CAD build for the part. Positions are in the model's coordinates, mm. Face numbers are marked on the shaded views. Give positions to 0.01 mm unless a question says otherwise; leave off trailing zeros. Loops run counter-clockwise (first coordinate to the right, second up) from the corner with the lowest first, then second, coordinate; pieces in that order, holes last.
Item 1: Drop flat-ended pins along their axis: P1, Ø1.5, axis at x = 9.5, y = 11, coming from the -Z side; P2, Ø4, axis at x = 17, z = 43.5, coming from the +Y side; P3, Ø8, axis at x = 14.5, y = 1, coming from the -Z side; P4, Ø7.5, axis at y = -19.19, z = -12.33, coming from the +X side. Give the stop position or say it passes through.
Item 2: Probe probe 1 along Z at (x, y) = (7, -18); probe 2 along Z at (x, y) = (2.75, -24) (3 decimals); probe 3 along Y at (x, z) = (15.5, -9). List the from-to ranges inside material, lowest first.
Item 3: Mould opens along Z. For the marked faces 1, 2, 3 and 4 say: released by +Z, released by -Z, zero draft, split by the parting line, or undercut.
Item 4: Saw through at B-B on x = 6. Give the cut face in (y, z).
Item 5: Saw through at A-A on z = 63. Give the cut face in (x, y).
Item 6: Saw through at C-C on y = -20.5. Give the cut face in (x, z), plus the area to 3 significant figures.
Item 7: Saw through at D-D on z = -11. Give the cut face in (x, y), plus the area to 3 significant figures.
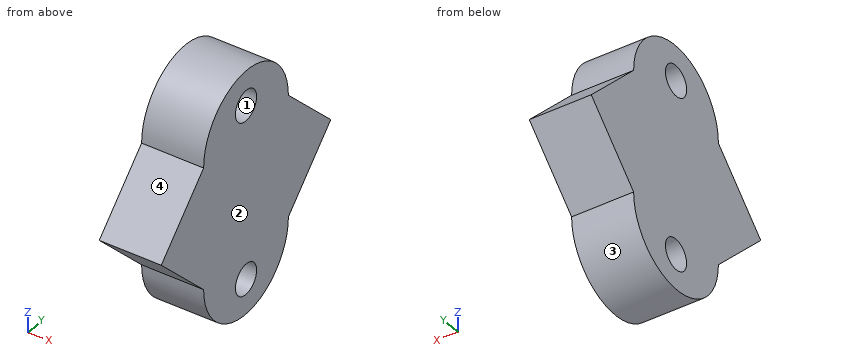
from build123d import *

# Parameters (mm, degrees)
F0_W     = 50.8
F0_H     = 50.8
F1_DEPTH = 25.4
F3_D     = 12.7


with BuildPart() as f1:
    # F0 (on Right) → F1 (new body)
    with BuildSketch(Plane.YZ):
        with BuildLine():
            ThreePointArc((6.2123674129, 49.3127632231), (-19.1876325871, 74.7127632231), (-44.5876325871, 49.3127632231))
            Line((-44.5876325871, 49.3127632231), (6.2123674129, 49.3127632231))
        make_face()
        with Locations((-19.1876325871, 23.9127632231)):
            Rectangle(F0_W, F0_H)
        Polygon((-44.5876325871, -1.4872367769), (-44.5876325871, 49.3127632231), (-69.9876325871, 23.9127632231), align=None)
        Polygon((31.6123674129, 23.9127632231), (6.2123674129, 49.3127632231), (6.2123674129, -1.4872367769), align=None)
        with BuildLine():
            Line((6.2123674129, -1.4872367769), (-44.5876325871, -1.4872367769))
            ThreePointArc((-44.5876325871, -1.4872367769), (-19.1876325871, -26.8872367769), (6.2123674129, -1.4872367769))
        make_face()
    extrude(amount=F1_DEPTH)

    # F3 (through all)
    with Locations(Plane.YZ.offset(25.4)):
        with Locations((-19.1876325871, 60.1578950882), (-19.1876325871, -12.3323686421)):
            Hole(F3_D / 2)


solid = f1.part
Results below:
1. P1: stops at z = 2.55
1. P2: stops at y = 14.03
1. P3: stops at z = -21.06
1. P4: passes through
2. probe 1: z = -26.86 to -18.57, -6.09 to 53.92, 66.4 to 74.68
2. probe 2: z = -26.427 to -16.475, -8.189 to 56.015, 64.301 to 74.253
2. probe 3: y = -43.45 to -24.59, -13.78 to 5.08
3. face 1: undercut
3. face 2: zero draft
3. face 3: released by -Z
3. face 4: released by +Z
4. outline: (-69.99, 23.91) - (-44.59, -1.49) arc R25.4 ccw to (6.21, -1.49) - (31.61, 23.91) - (6.21, 49.31) arc R25.4 ccw to (-44.59, 49.31) - close; hole circle Ø12.7 at (-19.19, -12.33); hole circle Ø12.7 at (-19.19, 60.16)
5. outline: (0, -40.58) - (25.4, -40.58) - (25.4, -24.87) - (0, -24.87) - close; (0, -13.51) - (25.4, -13.51) - (25.4, 2.21) - (0, 2.21) - close
6. outline: (0, -26.85) - (25.4, -26.85) - (25.4, -18.55) - (0, -18.55) - close; (0, -6.12) - (25.4, -6.12) - (25.4, 53.94) - (0, 53.94) - close; (0, 66.37) - (25.4, 66.37) - (25.4, 74.68) - (0, 74.68) - close
6. area: 1,950 mm2
7. outline: (0, -42.74) - (25.4, -42.74) - (25.4, -25.4) - (0, -25.4) - close; (0, -12.98) - (25.4, -12.98) - (25.4, 4.36) - (0, 4.36) - close
7. area: 881 mm2
